Can you work these out from the model? Positions are in its coordinate system, mm. Face numbers are marked on the shaded views. Coordinates: 2 decimals unless noted, no trailing zeros. Write each loop counter-clockwise with the first axis right and the second up, starting at its lowest first coordinate (ties: lowest second). Pieces come first, ordered by that corner, then holes. Notation, with made-up numbers: (46, 49) - (98, 49) arc R27 cw to (98, 78) - close; hole circle Ø8 at (69, -11). An arc over 180 degrees is marked (long way). Use one line per item in the form item = value. Start each with the question number.
(1) For pin 1 Ø1 at (y, z) = (-43, 40.5) entering from -X, with a flat end and sliding along its axis, tell me the tip position at first contact or that it passes through.
(2) If we section it at B-B on y = -43: Please give me the cut outline in (x, z).
(3) If we section it at C-C on z = 43: Please give me the cut outline in (x, y).
(4) If we section it at D-D on y = -59: Please give me the cut outline in (x, z), then the cut area to 3 significant figures.
(5) If we section it at A-A on x = -28: Please give me the cut outline in (y, z).
(6) If I drill on probe 1 along Y at (x, z) = (-39, 38); probe 2 along X at (y, z) = (-38.5, 48.5); probe 3 along X at (y, z) = (-34, 41.5), over which ranges is the centre line in solid material (lowest first)? Write a range as from..to.
(7) Thinking about a two-plate mould opening in X: for the marked faces 1, 2 and 3, which applies, pulls with the +X half, pulls with the -X half, needs draft (parallel to the pull), parting line crosses it, or undercut?
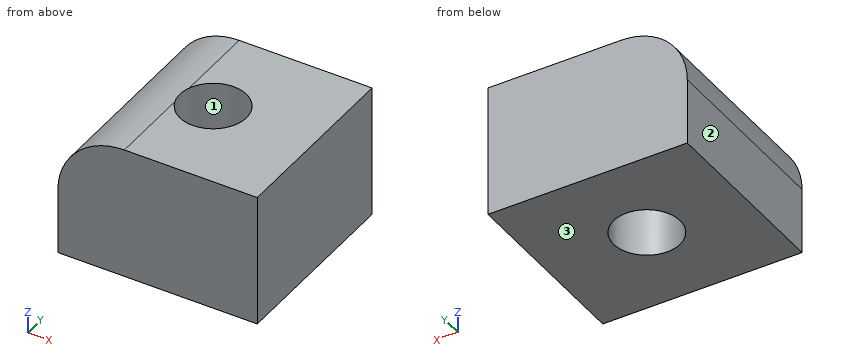
```python
from build123d import *

# Parameters (mm, degrees)
F1_DEPTH = 71.628
F2_R     = 12.7
F3_DEPTH = 50.801


with BuildPart() as f1:
    # F0 (on Front) → F1 (new body)
    with BuildSketch(Plane.XZ):
        with BuildLine():
            Line((-76.2, 0), (0, 0))
            Line((0, 0), (0, 50.8))
            Line((0, 50.8), (-50.8, 50.8))
            ThreePointArc((-50.8, 50.8), (-68.760512, 43.360512), (-76.2, 25.4))
            Line((-76.2, 25.4), (-76.2, 0))
        make_face()
    extrude(amount=F1_DEPTH)

    # F2 (on face) → F3 (cut, through all)
    with BuildSketch(Plane(origin=(0, 0, 0), x_dir=(1, 0, 0), z_dir=(0, 0, -1))):
        with Locations((-38.918827, 35.650235)):
            Circle(F2_R)
    extrude(amount=-F3_DEPTH, mode=Mode.SUBTRACT)


solid = f1.part
```
Reported:
q1.pin_1 = -71.58
q2.outline = (-76.2, 0) - (-49.28, 0) - (-49.28, 50.8) - (-50.8, 50.8) arc R25.4 ccw to (-76.2, 25.4) - close; (-28.56, 0) - (0, 0) - (0, 50.8) - (-28.56, 50.8) - close
q3.outline = (-69.11, -71.63) - (0, -71.63) - (0, 0) - (-69.11, 0) - close; hole circle Ø25.4 at (-38.92, -35.65)
q4.outline = (-76.2, 0) - (0, 0) - (0, 50.8) - (-50.8, 50.8) arc R25.4 ccw to (-76.2, 25.4) - close
q4.area = 3,730 mm2
q5.outline = (-71.63, 0) - (-42.14, 0) - (-42.14, 50.8) - (-71.63, 50.8) - close; (-29.16, 0) - (0, 0) - (0, 50.8) - (-29.16, 50.8) - close
q6.probe_1 = -71.63..-48.35, -22.95..0
q6.probe_2 = -61.36..-51.29, -26.54..0
q6.probe_3 = -70.45..-51.51, -26.33..0
q7.face_1 = undercut
q7.face_2 = pulls with the -X half
q7.face_3 = needs draft
